Input: part model. Units: mm. Frame: model coordinates. A direction names the side the tool comes from. Coordinates: 2 decimals unless noted, no trailing zeros. Order: outer loops, then holes, each group sorted by start corner. A loop starts at its lowest first (then second) coordinate and runs counter-clockwise, first axis right, second up. Notation, with made-up numbers: M -30.5,-12.75 L 22.5,-12.75 A23 ccw 22.5,23.25 Z; hole C -31.75,1.5 d1. An arc over 180 degrees is marked long. Answer in a Markdown table with one row per item.
from build123d import *

# Parameters (mm, degrees)
BOSS_EXTRUDE1_DEPTH     = 20
FILLET1_R               = 15
CUT_EXTRUDE1_DEPTH      = 56.162909807
CUT_EXTRUDE1_DEPTH_BACK = 56.162909807
SKETCH3_R               = 4.25
SKETCH4_R               = 3
CUT_EXTRUDE2_DEPTH      = 14


with BuildPart() as part:
    # Sketch1 → Boss-Extrude1 (new, symmetric)
    with BuildSketch(Plane.XY):
        with BuildLine():
            Line((-25, 0), (-33.49547145, 0))
            Line((-33.49547145, 0), (-23, 35))
            Line((-23, 35), (-23, 39))
            Line((-23, 39), (23, 39))
            Line((23, 39), (23, 35))
            Line((23, 35), (33.49547145, 0))
            Line((33.49547145, 0), (25, 0))
            ThreePointArc((25, 0), (0, 25), (-25, 0))
        make_face()
    extrude(amount=BOSS_EXTRUDE1_DEPTH, both=True)

    # Fillet1
    fillet1_edges = [part.edges().sort_by_distance(p)[0] for p in [
        (-29.247735725, 0, 20),
        (29.247735725, 0, 20),
        (29.247735725, 0, -20),
        (-29.247735725, 0, -20),
    ]]
    fillet(fillet1_edges, radius=FILLET1_R)

    # Sketch3 → Cut-Extrude1 (cut, two sides: drawn at the far end of the back side and taken through both)
    with BuildSketch(Plane(origin=(0, 0, 0), x_dir=(0, 0, -1), z_dir=(1, 0, 0)).offset(-CUT_EXTRUDE1_DEPTH_BACK)):
        with Locations((0, 12)):
            Circle(SKETCH3_R)
    extrude(amount=CUT_EXTRUDE1_DEPTH + CUT_EXTRUDE1_DEPTH_BACK, mode=Mode.SUBTRACT)

    # Sketch4 → Cut-Extrude2 (cut)
    with BuildSketch(Plane(origin=(0, 39, 0), x_dir=(1, 0, 0), z_dir=(0, 1, 0))):
        with Locations(Location((-12, 0, 0), (0, 0, 270))):
            Circle(SKETCH4_R)
        with Locations(Location((12, 0, 0), (0, 0, 270))):
            Circle(SKETCH4_R)
    extrude(amount=-CUT_EXTRUDE2_DEPTH, mode=Mode.SUBTRACT)


solid = part.part
1) Mould query, pull axis Y, two halves, no side actions, for faces 5 (the face through (12, 25, 0)), 6 (the face through (-28.34, 4.28, -15.49)), 7 (the face through (-25.173, 16.214, 0.553)). Classes: +Y half, -Y half, draft (parallel to the pull), parting line (faces both ways), or undercut.
Resolved:
| item | result |
|---|---|
| face 5 | +Y half |
| face 6 | -Y half |
| face 7 | undercut |
2) Reachability of faces 1 (the face through (-23, 37, 0)), 2 (the face through (24.987, 16.214, 0.553)), 3 (the face through (-14.662, 32.098, 1.384)), 4 (the face through (23, 37, 0)) from +Z, -Z, +X, -X, +Y, -Y: full face, straight path, thin tool, end or side. Return the list, or none.
Resolved:
| item | result |
|---|---|
| face 1 | +Z, -Z, -X, +Y |
| face 2 | +X, -X |
| face 3 | +Y |
| face 4 | +Z, -Z, +X, +Y |
3) Contact query for flat-ended pins moving along their axis: pin 1 (5 mm diameter, centred on y = 34, z = -13, fed in from -X); pin 2 (5 mm diameter, centred on y = 15, z = 6, fed in from +X); pin 3 (1 mm diameter, centred on y = 17.5, z = -1, fed in from +X); pin 4 (7.5 mm diameter, centred on y = 12, z = 0, fed in from +X). Output: stop coordinate, or through.
Resolved:
| item | result |
|---|---|
| pin 1 | stops at x = -24.05 |
| pin 2 | stops at x = 29.75 |
| pin 3 | stops at x = 28.4 |
| pin 4 | passes through |
4) Cut plane D-D, the plane x = -27. Output: boundary loops of the cut face in (y, z).
Resolved:
| item | result |
|---|---|
| outline | M 0,-5 A15 ccw 15,-20 L 21.66,-20 L 21.66,20 L 15,20 A15 ccw 0,5 Z; hole C 12,0 d8.5 |
5) Material intervals for probe 1 along X at (y, z) = (31.75, 0); probe 2 along X at (y, z) = (27, 1); probe 3 along X at (y, z) = (4, 0.5), sorted ascending.
Resolved:
| item | result |
|---|---|
| probe 1 | x = -23.97 to -15, -9 to 9, 15 to 23.97 |
| probe 2 | x = -25.4 to -14.83, -9.17 to 9.17, 14.83 to 25.4 |
| probe 3 | x = -32.3 to -24.68, 24.68 to 32.3 |
6) Cut plane C-C, the plane y = 17.5. Output: boundary loops of the cut face in (x, z), and give its area (3 significant figures).
Resolved:
| item | result |
|---|---|
| outline | M -28.25,-20 L -17.85,-20 L -17.85,20 L -28.25,20 Z; M 17.85,-20 L 28.25,-20 L 28.25,20 L 17.85,20 Z |
| area | 832 mm2 |
7) Cut plane B-B, the plane y = 11. Output: boundary loops of the cut face in (x, z), and give its area (3 significant figures).
Resolved:
| item | result |
|---|---|
| outline | M -30.2,-19.46 L -22.45,-19.46 L -22.45,-4.13 L -30.2,-4.13 Z; M -30.2,4.13 L -22.45,4.13 L -22.45,19.46 L -30.2,19.46 Z; M 22.45,-19.46 L 30.2,-19.46 L 30.2,-4.13 L 22.45,-4.13 Z; M 22.45,4.13 L 30.2,4.13 L 30.2,19.46 L 22.45,19.46 Z |
| area | 475 mm2 |
8) Cut plane A-A, the plane z = 0. Output: boundary loops of the cut face in (x, y).
Resolved:
| item | result |
|---|---|
| outline | M -33.5,0 L -25,0 A25 cw -23.77,7.75 L -31.17,7.75 Z; M -28.62,16.25 L -19,16.25 A25 cw 19,16.25 L 28.62,16.25 L 23,35 L 23,39 L 15,39 L 15,25 L 9,25 L 9,39 L -9,39 L -9,25 L -15,25 L -15,39 L -23,39 L -23,35 Z; M 23.77,7.75 A25 cw 25,0 L 33.5,0 L 31.17,7.75 Z |
